Can you work these out from the drawing? Everything is in mm from the part's minimum corner. Coordinates: 2 decimals unless noted, no trailing zeros. Order: outer loops, then holes, each group sorted by start corner. A loop starts at its lowest first (then second) coordinate and runs counter-clockwise, first axis right, second up. Notation, with made-up numbers: (-29, 10) - (3, 10) arc R27 cw to (3, 42) - close; hole circle Ø9 at (-19.5, 0.5). An arc over 180 degrees is marked (long way). Answer as CSV lines item,"result". Start each with the question number.
Q1. I need wall thicknesses on line 1 (Z direction, x = 2, y = 0.95); line 2 (Z direction, x = 0.75, y = 0.8); line 3 (Y direction, x = 5, z = 0.3). Which ranges of each line are inside material? Lowest first, please.
Q2. Suppose I cut it at A-A (x = 7). Please give me the cut outline in (y, z), then the cut area to 3 significant figures.
Q3. Suppose I cut it at B-B (y = 0.8). Please give me the cut outline in (x, z), then the cut area to 3 significant figures.
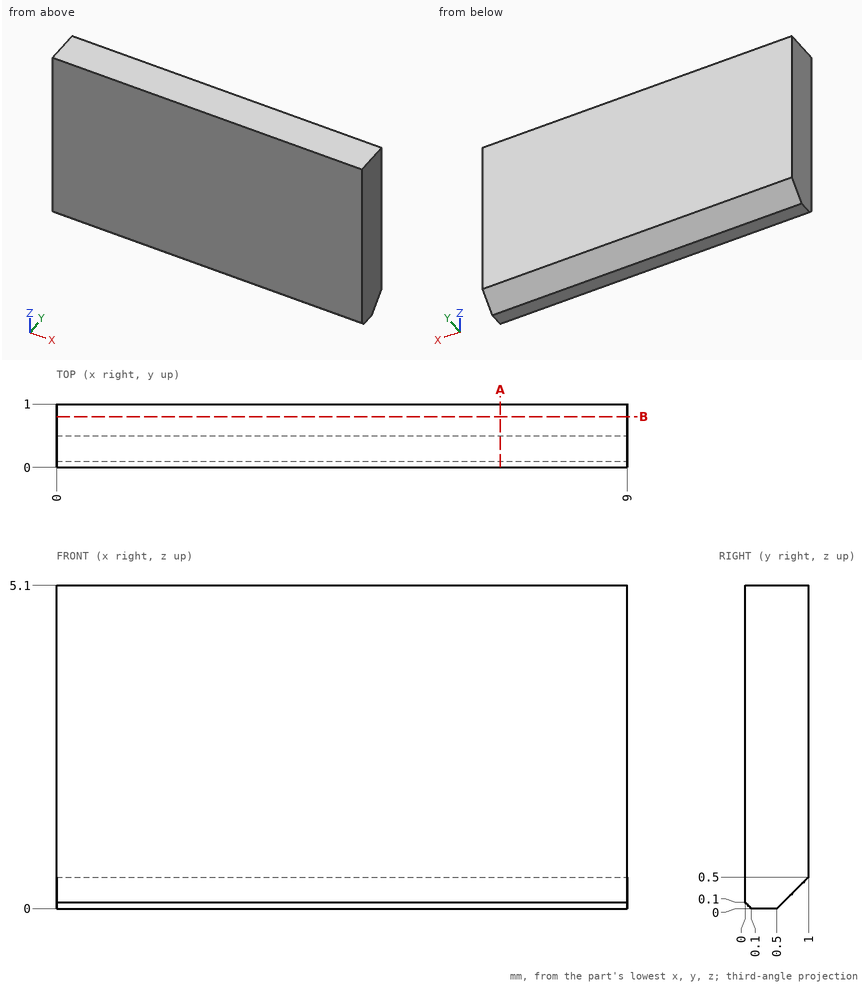
Here are the results:
1,line 1,"z = 0.45 to 5.1"
1,line 2,"z = 0.3 to 5.1"
1,line 3,"y = 0 to 0.8"
2,outline,"(0, 0.1) - (0.1, 0) - (0.5, 0) - (1, 0.5) - (1, 5.1) - (0, 5.1) - close"
2,area,"4.97 mm²"
3,outline,"(0, 0.3) - (9, 0.3) - (9, 5.1) - (0, 5.1) - close"
3,area,"43.2 mm²"
